Answer from the drawing. Dimensions are ordinates in mm from the lowest x, y and z of the part. A direction names the side the tool comes from. Round coordinates to 2 decimals unless told otherwise and drop trailing zeros. Order: outer loops, then holes, each group sorted by start corner. A loop starts at its lowest first (then second) coordinate and runs counter-clockwise, first axis right, second up. Notation, with made-up numbers: M -33,22 L -19,22 A18 cw -19,47 Z; hole C 22.25,51.5 d8. An arc over 180 degrees is marked long. Answer as a JSON object with one key per item and string values. Group by question number.
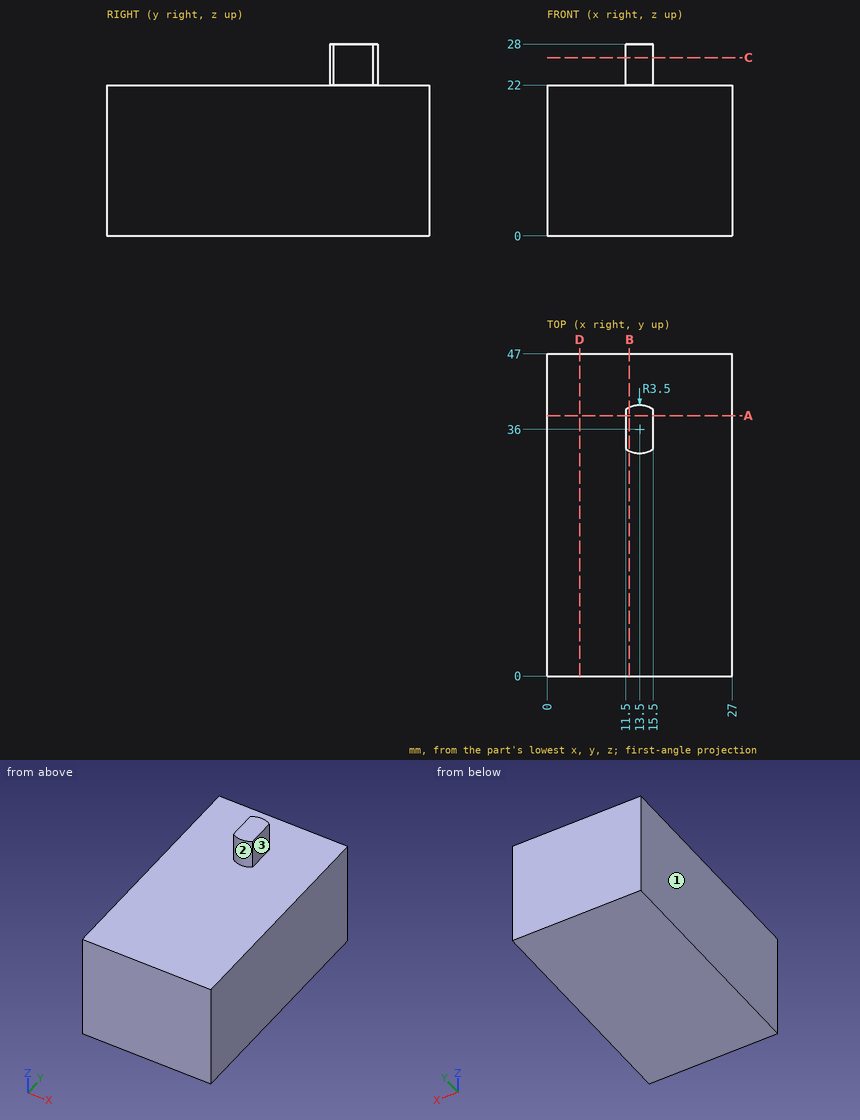
Item 1: Find section B-B (x = 12). Give the vertices of the cut face in (y, z).
Item 2: Find section A-A (y = 38). Give the vertices of the cut face in (x, z).
Item 3: Consider L1, parallel to Z at x = 13.25, y = 40. Determine where the line is inside the solid, lowest interval first.
Item 4: Each of these flat-tipped pins is pushed along its axis until it touches: pin 1 (1 mm diameter, centred on x = 9.5, y = 14, fed in from +Z); pin 2 (8 mm diameter, centred on x = 17.5, y = 7.5, fed in from -Z); pin 3 (4.5 mm diameter, centred on y = 36, z = 25.5, fed in from -X); pin 4 (1.7 mm diameter, centred on y = 34.5, z = 23.5, fed in from +X). Where does it stop, or does it pass through?
Item 5: Find section D-D (x = 4.75). Give the vertices of the cut face in (y, z).
Item 6: Find section C-C (z = 26). Give the vertices of the cut face in (x, y).
Item 7: A tool of negligible diameter and unlimited length cuts with its end or side. For the marked faces 1, 2 and 3, from which of +Z, -Z, +X, -X, +Y, -Y can it reach the whole face along a straight path? Write none if from no direction.
Responses:
{
 "1": {"outline": "M 0,0 L 47,0 L 47,22 L 39.16,22 L 39.16,28 L 32.84,28 L 32.84,22 L 0,22 Z"},
 "2": {"outline": "M 0,0 L 27,0 L 27,22 L 15.5,22 L 15.5,28 L 11.5,28 L 11.5,22 L 0,22 Z"},
 "3": {"L1": "z = 0 to 22"},
 "4": {"pin 1": "stops at z = 22", "pin 2": "stops at z = 0", "pin 3": "stops at x = 11.5", "pin 4": "stops at x = 15.5"},
 "5": {"outline": "M 0,0 L 47,0 L 47,22 L 0,22 Z"},
 "6": {"outline": "M 11.5,33.13 A3.5 ccw 15.5,33.13 L 15.5,38.87 A3.5 ccw 11.5,38.87 Z"},
 "7": {"face 1": "+Z, -Z, -X, +Y, -Y", "face 2": "+Z, -Y", "face 3": "+Z, +X, +Y, -Y"}
}
